Here's the drawing with two shaded views (mm, measured from the low corner). I have some questions. Round coordinates to 2 decimals unless told otherwise and drop trailing zeros. Loops run counter-clockwise (first coordinate to the right, second up) from the corner with the lowest first, then second, coordinate; pieces in that order, holes last. Notation, with made-up numbers: (17, 83.5) -> (54, 83.5) arc R21 cw to (54, 104.5) -> close; hole circle Ø3 at (38, -38.75). An arc over 180 degrees is marked (long way). Write each question's results on one line, items separated by ' | '.
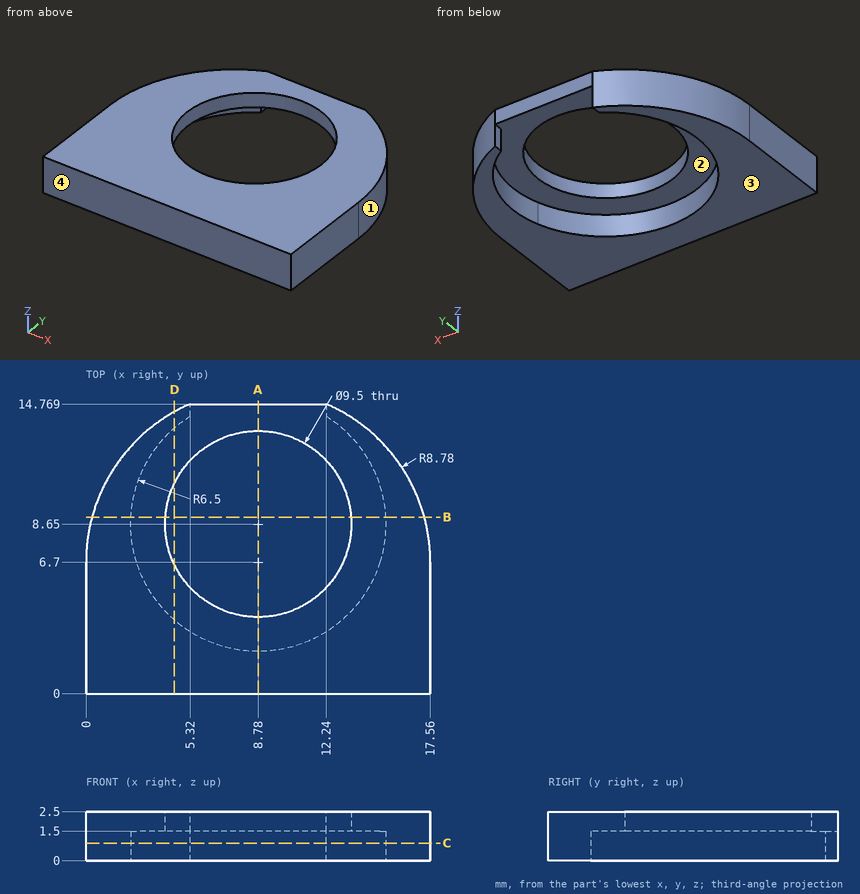
1. If we section it at A-A (x = 8.78): List the corners of the cut face in (y, z) for me.
Final values:
outline: (0, 0) -> (2.15, 0) -> (2.15, 1.5) -> (3.9, 1.5) -> (3.9, 2.5) -> (0, 2.5) -> close; (13.4, 1.5) -> (14.77, 1.5) -> (14.77, 2.5) -> (13.4, 2.5) -> close
2. We'd pull the mould along Y, two halves only. Please class the marked faces 1, 2, 3 and 4: pulls with the +Y half, pulls with the -Y half, needs draft (parallel to the pull), parting line crosses it, or undercut.
Final values:
face 1: pulls with the +Y half | face 2: undercut | face 3: needs draft | face 4: pulls with the -Y half
3. If we section it at B-B (y = 9): List the corners of the cut face in (x, z) for me, then the cut area to 3 significant figures.
Final values:
outline: (0.31, 0) -> (2.29, 0) -> (2.29, 1.5) -> (4.04, 1.5) -> (4.04, 2.5) -> (0.31, 2.5) -> close; (13.52, 1.5) -> (15.27, 1.5) -> (15.27, 0) -> (17.25, 0) -> (17.25, 2.5) -> (13.52, 2.5) -> close | area: 13.4 mm2
4. Please list where these lines run through material, in increasing order: line 1 (Y direction, x = 8.78, z = 1.75); line 2 (Y direction, x = 9, z = 1.2); line 3 (X direction, y = 14.25, z = 1.25) (1 decimal). Write a range as from..to.
Final values:
line 1: 0..3.9, 13.4..14.77 | line 2: 0..2.15 | line 3: 4.3..5.3, 12.2..13.3
5. If we section it at D-D (x = 4.5): List the corners of the cut face in (y, z) for me.
Final values:
outline: (0, 0) -> (3.76, 0) -> (3.76, 1.5) -> (6.59, 1.5) -> (6.59, 2.5) -> (0, 2.5) -> close; (10.71, 1.5) -> (13.54, 1.5) -> (13.54, 0) -> (14.37, 0) -> (14.37, 2.5) -> (10.71, 2.5) -> close
6. If we section it at C-C (z = 0.9): List the corners of the cut face in (x, y) for me, then the cut area to 3 significant figures.
Final values:
outline: (0, 0) -> (17.56, 0) -> (17.56, 6.7) arc R8.78 ccw to (12.24, 14.77) -> (12.24, 14.15) arc R6.5 cw (long way) to (5.32, 14.15) -> (5.32, 14.77) arc R8.78 ccw to (0, 6.7) -> close | area: 103 mm2
7. Will these pins go through, and if not, where does the flat tip stop? pin 1 (0.7 mm diameter, centred on y = 14.5, z = 1, fed in from -X) (1 decimal); pin 2 (1 mm diameter, centred on y = 11, z = 1, fed in from -X) (1 decimal); pin 3 (4 mm diameter, centred on x = 6.5, y = 8.5, fed in from -Z).
Final values:
pin 1: x = 4.1 | pin 2: x = 0.9 | pin 3: through
